from build123d import *

# Parameters (mm, degrees)
SKETCH1_W                   = 14.4272
SKETCH1_H                   = 11.43
CUT_EXTRUDE1_DEPTH          = 22.666423328
CUT_EXTRUDE2_DEPTH          = 22.666423328
CUT_EXTRUDE3_DEPTH          = 22.666423328
CUT_EXTRUDE4_DEPTH          = 22.666423328
CUT_EXTRUDE5_DEPTH          = 22.666423328
CUT_EXTRUDE6_DEPTH          = 22.666423328
CUT_EXTRUDE7_DEPTH          = 22.666423328
CUT_EXTRUDE8_DEPTH          = 22.666423328
CUT_EXTRUDE9_DEPTH          = 22.666423328
CUT_EXTRUDE10_DEPTH         = 22.666423328
CUT_EXTRUDE11_DEPTH         = 22.666423328
CUT_EXTRUDE12_DEPTH         = 22.589197779
CUT_EXTRUDE13_DEPTH         = 22.589197779
CUT_EXTRUDE14_DEPTH         = 22.589197779
CUT_EXTRUDE15_DEPTH         = 22.589197779
CUT_EXTRUDE16_DEPTH         = 22.511694997
F_1_4_0_25_DIAMETER_HOLE1_D = 12.7


with BuildPart() as part:
    # Sketch1 → Revolve1 (revolve)
    with BuildSketch(Plane(origin=(0, 0, 0), x_dir=(-1, 0, 0), z_dir=(0, 0, -1)), mode=Mode.PRIVATE) as revolve1_sk:
        with Locations((-7.2136, 5.715)):
            Rectangle(SKETCH1_W, SKETCH1_H)
    revolve(revolve1_sk.sketch.rotate(Axis((14.4272, 0, 0), (-1, 0, 0)), 270), axis=Axis((14.4272, 0, 0), (-1, 0, 0)))

    # Sketch2 → Cut-Extrude1 (cut, through all)
    with BuildSketch(Plane(origin=(14.4272, 0, 0), x_dir=(0, 0, -1), z_dir=(1, 0, 0))):
        with BuildLine():
            ThreePointArc((9.270604538, 6.685865052), (8.082230509, 8.082230509), (6.685865052, 9.270604538))
            ThreePointArc((6.685865052, 9.270604538), (6.338531077, 7.823071544), (5.493243318, 6.597722098))
            ThreePointArc((5.493243318, 6.597722098), (6.070653138, 6.070653138), (6.597722098, 5.493243318))
            ThreePointArc((6.597722098, 5.493243318), (7.823071544, 6.338531077), (9.270604538, 6.685865052))
        make_face()
    extrude(amount=-CUT_EXTRUDE1_DEPTH, mode=Mode.SUBTRACT)

    # Sketch3 → Cut-Extrude2 (cut, through all)
    with BuildSketch(Plane(origin=(14.4272, 0, 0), x_dir=(0, 0, -1), z_dir=(1, 0, 0))):
        with BuildLine():
            ThreePointArc((11.123491573, 2.629227114), (10.559943057, 4.374071632), (9.724640644, 6.006352))
            ThreePointArc((9.724640644, 6.006352), (8.849798999, 4.801924852), (7.599934007, 3.9933272))
            ThreePointArc((7.599934007, 3.9933272), (7.931690563, 3.285413804), (8.197673616, 2.550256131))
            ThreePointArc((8.197673616, 2.550256131), (9.65322651, 2.862279258), (11.123491573, 2.629227114))
        make_face()
    extrude(amount=-CUT_EXTRUDE2_DEPTH, mode=Mode.SUBTRACT)

    # Sketch4 → Cut-Extrude3 (cut, through all)
    with BuildSketch(Plane(origin=(14.4272, 0, 0), x_dir=(0, 0, -1), z_dir=(1, 0, 0))):
        with BuildLine():
            ThreePointArc((11.282927851, -1.827686818), (11.43, 0), (11.282927851, 1.827686818))
            ThreePointArc((11.282927851, 1.827686818), (10.013765246, 1.049728631), (8.549603637, 0.780984435))
            ThreePointArc((8.549603637, 0.780984435), (8.5852, 0), (8.549603637, -0.780984435))
            ThreePointArc((8.549603637, -0.780984435), (10.013765246, -1.049728631), (11.282927851, -1.827686818))
        make_face()
    extrude(amount=-CUT_EXTRUDE3_DEPTH, mode=Mode.SUBTRACT)

    # Sketch5 → Cut-Extrude4 (cut, through all)
    with BuildSketch(Plane(origin=(14.4272, 0, 0), x_dir=(0, 0, -1), z_dir=(1, 0, 0))):
        with BuildLine():
            ThreePointArc((9.724640644, -6.006352), (10.559943057, -4.374071632), (11.123491573, -2.629227114))
            ThreePointArc((11.123491573, -2.629227114), (9.65322651, -2.862279258), (8.197673616, -2.550256131))
            ThreePointArc((8.197673616, -2.550256131), (7.931690563, -3.285413804), (7.599934007, -3.9933272))
            ThreePointArc((7.599934007, -3.9933272), (8.849798999, -4.801924852), (9.724640644, -6.006352))
        make_face()
    extrude(amount=-CUT_EXTRUDE4_DEPTH, mode=Mode.SUBTRACT)

    # Sketch6 → Cut-Extrude5 (cut, through all)
    with BuildSketch(Plane(origin=(14.4272, 0, 0), x_dir=(0, 0, -1), z_dir=(1, 0, 0))):
        with BuildLine():
            ThreePointArc((6.685865052, -9.270604538), (8.082230509, -8.082230509), (9.270604538, -6.685865052))
            ThreePointArc((9.270604538, -6.685865052), (7.823071544, -6.338531077), (6.597722098, -5.493243318))
            ThreePointArc((6.597722098, -5.493243318), (6.070653138, -6.070653138), (5.493243318, -6.597722098))
            ThreePointArc((5.493243318, -6.597722098), (6.338531077, -7.823071544), (6.685865052, -9.270604538))
        make_face()
    extrude(amount=-CUT_EXTRUDE5_DEPTH, mode=Mode.SUBTRACT)

    # Sketch7 → Cut-Extrude6 (cut, through all)
    with BuildSketch(Plane(origin=(14.4272, 0, 0), x_dir=(0, 0, -1), z_dir=(1, 0, 0))):
        with BuildLine():
            ThreePointArc((2.629227114, -11.123491573), (4.374071632, -10.559943057), (6.006352, -9.724640644))
            ThreePointArc((6.006352, -9.724640644), (4.801924852, -8.849798999), (3.9933272, -7.599934007))
            ThreePointArc((3.9933272, -7.599934007), (3.285413804, -7.931690563), (2.550256131, -8.197673616))
            ThreePointArc((2.550256131, -8.197673616), (2.862279258, -9.65322651), (2.629227114, -11.123491573))
        make_face()
    extrude(amount=-CUT_EXTRUDE6_DEPTH, mode=Mode.SUBTRACT)

    # Sketch8 → Cut-Extrude7 (cut, through all)
    with BuildSketch(Plane(origin=(14.4272, 0, 0), x_dir=(0, 0, -1), z_dir=(1, 0, 0))):
        with BuildLine():
            ThreePointArc((-1.827686818, -11.282927851), (0, -11.43), (1.827686818, -11.282927851))
            ThreePointArc((1.827686818, -11.282927851), (1.049728631, -10.013765246), (0.780984435, -8.549603637))
            ThreePointArc((0.780984435, -8.549603637), (0, -8.5852), (-0.780984435, -8.549603637))
            ThreePointArc((-0.780984435, -8.549603637), (-1.049728631, -10.013765246), (-1.827686818, -11.282927851))
        make_face()
    extrude(amount=-CUT_EXTRUDE7_DEPTH, mode=Mode.SUBTRACT)

    # Sketch9 → Cut-Extrude8 (cut, through all)
    with BuildSketch(Plane(origin=(14.4272, 0, 0), x_dir=(0, 0, -1), z_dir=(1, 0, 0))):
        with BuildLine():
            ThreePointArc((-6.006352, -9.724640644), (-4.374071632, -10.559943057), (-2.629227114, -11.123491573))
            ThreePointArc((-2.629227114, -11.123491573), (-2.862279258, -9.65322651), (-2.550256131, -8.197673616))
            ThreePointArc((-2.550256131, -8.197673616), (-3.285413804, -7.931690563), (-3.9933272, -7.599934007))
            ThreePointArc((-3.9933272, -7.599934007), (-4.801924852, -8.849798999), (-6.006352, -9.724640644))
        make_face()
    extrude(amount=-CUT_EXTRUDE8_DEPTH, mode=Mode.SUBTRACT)

    # Sketch10 → Cut-Extrude9 (cut, through all)
    with BuildSketch(Plane(origin=(14.4272, 0, 0), x_dir=(0, 0, -1), z_dir=(1, 0, 0))):
        with BuildLine():
            ThreePointArc((-9.270604538, -6.685865052), (-8.082230509, -8.082230509), (-6.685865052, -9.270604538))
            ThreePointArc((-6.685865052, -9.270604538), (-6.338531077, -7.823071544), (-5.493243318, -6.597722098))
            ThreePointArc((-5.493243318, -6.597722098), (-6.070653138, -6.070653138), (-6.597722098, -5.493243318))
            ThreePointArc((-6.597722098, -5.493243318), (-7.823071544, -6.338531077), (-9.270604538, -6.685865052))
        make_face()
    extrude(amount=-CUT_EXTRUDE9_DEPTH, mode=Mode.SUBTRACT)

    # Sketch11 → Cut-Extrude10 (cut, through all)
    with BuildSketch(Plane(origin=(14.4272, 0, 0), x_dir=(0, 0, -1), z_dir=(1, 0, 0))):
        with BuildLine():
            ThreePointArc((-11.123491573, -2.629227114), (-10.559943057, -4.374071632), (-9.724640644, -6.006352))
            ThreePointArc((-9.724640644, -6.006352), (-8.849798999, -4.801924852), (-7.599934007, -3.9933272))
            ThreePointArc((-7.599934007, -3.9933272), (-7.931690563, -3.285413804), (-8.197673616, -2.550256131))
            ThreePointArc((-8.197673616, -2.550256131), (-9.65322651, -2.862279258), (-11.123491573, -2.629227114))
        make_face()
    extrude(amount=-CUT_EXTRUDE10_DEPTH, mode=Mode.SUBTRACT)

    # Sketch12 → Cut-Extrude11 (cut, through all)
    with BuildSketch(Plane(origin=(14.4272, 0, 0), x_dir=(0, 0, -1), z_dir=(1, 0, 0))):
        with BuildLine():
            ThreePointArc((-11.282927851, 1.827686818), (-11.43, 0), (-11.282927851, -1.827686818))
            ThreePointArc((-11.282927851, -1.827686818), (-10.013765246, -1.049728631), (-8.549603637, -0.780984435))
            ThreePointArc((-8.549603637, -0.780984435), (-8.5852, 0), (-8.549603637, 0.780984435))
            ThreePointArc((-8.549603637, 0.780984435), (-10.013765246, 1.049728631), (-11.282927851, 1.827686818))
        make_face()
    extrude(amount=-CUT_EXTRUDE11_DEPTH, mode=Mode.SUBTRACT)

    # Sketch13 → Cut-Extrude12 (cut, through all)
    with BuildSketch(Plane(origin=(14.4272, 0, 0), x_dir=(0, 0, -1), z_dir=(1, 0, 0))):
        with BuildLine():
            ThreePointArc((-9.724640644, 6.006352), (-10.559943057, 4.374071632), (-11.123491573, 2.629227114))
            ThreePointArc((-11.123491573, 2.629227114), (-9.65322651, 2.862279258), (-8.197673616, 2.550256131))
            ThreePointArc((-8.197673616, 2.550256131), (-7.931690563, 3.285413804), (-7.599934007, 3.9933272))
            ThreePointArc((-7.599934007, 3.9933272), (-8.849798999, 4.801924852), (-9.724640644, 6.006352))
        make_face()
    extrude(amount=-CUT_EXTRUDE12_DEPTH, mode=Mode.SUBTRACT)

    # Sketch14 → Cut-Extrude13 (cut, through all)
    with BuildSketch(Plane(origin=(14.4272, 0, 0), x_dir=(0, 0, -1), z_dir=(1, 0, 0))):
        with BuildLine():
            ThreePointArc((-6.685865052, 9.270604538), (-8.082230509, 8.082230509), (-9.270604538, 6.685865052))
            ThreePointArc((-9.270604538, 6.685865052), (-7.823071544, 6.338531077), (-6.597722098, 5.493243318))
            ThreePointArc((-6.597722098, 5.493243318), (-6.070653138, 6.070653138), (-5.493243318, 6.597722098))
            ThreePointArc((-5.493243318, 6.597722098), (-6.338531077, 7.823071544), (-6.685865052, 9.270604538))
        make_face()
    extrude(amount=-CUT_EXTRUDE13_DEPTH, mode=Mode.SUBTRACT)

    # Sketch15 → Cut-Extrude14 (cut, through all)
    with BuildSketch(Plane(origin=(14.4272, 0, 0), x_dir=(0, 0, -1), z_dir=(1, 0, 0))):
        with BuildLine():
            ThreePointArc((-2.629227114, 11.123491573), (-4.374071632, 10.559943057), (-6.006352, 9.724640644))
            ThreePointArc((-6.006352, 9.724640644), (-4.801924852, 8.849798999), (-3.9933272, 7.599934007))
            ThreePointArc((-3.9933272, 7.599934007), (-3.285413804, 7.931690563), (-2.550256131, 8.197673616))
            ThreePointArc((-2.550256131, 8.197673616), (-2.862279258, 9.65322651), (-2.629227114, 11.123491573))
        make_face()
    extrude(amount=-CUT_EXTRUDE14_DEPTH, mode=Mode.SUBTRACT)

    # Sketch16 → Cut-Extrude15 (cut, through all)
    with BuildSketch(Plane(origin=(14.4272, 0, 0), x_dir=(0, 0, -1), z_dir=(1, 0, 0))):
        with BuildLine():
            ThreePointArc((1.827686818, 11.282927851), (0, 11.43), (-1.827686818, 11.282927851))
            ThreePointArc((-1.827686818, 11.282927851), (-1.049728631, 10.013765246), (-0.780984435, 8.549603637))
            ThreePointArc((-0.780984435, 8.549603637), (0, 8.5852), (0.780984435, 8.549603637))
            ThreePointArc((0.780984435, 8.549603637), (1.049728631, 10.013765246), (1.827686818, 11.282927851))
        make_face()
    extrude(amount=-CUT_EXTRUDE15_DEPTH, mode=Mode.SUBTRACT)

    # Sketch17 → Cut-Extrude16 (cut, through all)
    with BuildSketch(Plane(origin=(14.4272, 0, 0), x_dir=(0, 0, -1), z_dir=(1, 0, 0))):
        with BuildLine():
            ThreePointArc((6.006352, 9.724640644), (4.374071632, 10.559943057), (2.629227114, 11.123491573))
            ThreePointArc((2.629227114, 11.123491573), (2.862279258, 9.65322651), (2.550256131, 8.197673616))
            ThreePointArc((2.550256131, 8.197673616), (3.285413804, 7.931690563), (3.9933272, 7.599934007))
            ThreePointArc((3.9933272, 7.599934007), (4.801924852, 8.849798999), (6.006352, 9.724640644))
        make_face()
    extrude(amount=-CUT_EXTRUDE16_DEPTH, mode=Mode.SUBTRACT)

    # 1/4 (0.25) Diameter Hole1 (through all)
    with Locations(Plane(origin=(14.4272, 0, 0), x_dir=(0, 0, -1), z_dir=(1, 0, 0))):
        with Locations((0, 0)):
            Hole(F_1_4_0_25_DIAMETER_HOLE1_D / 2)


solid = part.part
The model under review builds one solid part; all positions refer to its coordinate system, in mm. A direction names the side the tool comes from. Coordinates: 2 decimals unless noted, no trailing zeros. Write each loop counter-clockwise with the first axis right and the second up, starting at its lowest first coordinate (ties: lowest second). Pieces come first, ordered by that corner, then holes. Notation, with made-up numbers: (62, 32.25) - (104, 32.25) arc R22 cw to (104, 63.25) - close; hole circle Ø9 at (5.25, -3.5). An arc over 180 degrees is marked (long way). Answer as CSV lines item,"result".
(1) Mouldability with a two-part tool opening along Y and no side actions: class faces 1 (the cylindrical face through (7.113, 2.224, 11.211)), 2 (the cylindrical face through (7.315, -2.863, -9.674)), 3 (the flat face through (14.427, 5, 5)) as pulls with the +Y half, pulls with the -Y half, needs draft (parallel to the pull), parting line crosses it, or undercut.
Data:
face 1,"pulls with the +Y half"
face 2,"undercut"
face 3,"needs draft"
(2) For line 1 along Y through (x, z) = (6.5, 0); line 2 along Y through (x, z) = (10.75, 9); line 3 along Y through (x, z) = (6.75, -4.5), list the stretches that pass through material, from the lowest coordinate up. Write a range as [from, to].
Data:
line 1,"y = [-8.59, -6.35], [6.35, 8.59]"
line 2,"y = [-6.66, -4.95], [-2.79, -0.8], [0.8, 2.79], [4.95, 6.66]"
line 3,"y = [-8.49, -4.48], [4.48, 8.49]"
(3) We need section C-C (y = 7). Give the boundary of the cut face in (x, z).
Data:
outline,"(0, -5.85) - (14.43, -5.85) - (14.43, 5.85) - (0, 5.85) - close"
(4) We need section A-A (y = 0). Give the boundary of the cut face in (x, z), plus the area to 3 significant figures.
Data:
outline,"(0, -8.59) - (14.43, -8.59) - (14.43, -6.35) - (0, -6.35) - close; (0, 6.35) - (14.43, 6.35) - (14.43, 8.59) - (0, 8.59) - close"
area,"64.5 mm2"
(5) Tool access review of faces 4 (the cylindrical face through (7.315, 3.296, -7.927)), 5 (the cylindrical face through (7.315, -0.011, 8.585)): name each direction out of +Z, -Z, +X, -X, +Y, -Y from which nothing blocks a thin tool from reaching the whole face with its end or side.
Data:
face 4,"+X, -X"
face 5,"+Z, +X, -X"
(6) Clearance check with flat-ended pins moving along their axes: pin 1 Ø1 at (y, z) = (-3.5, -7.5) entering from -X; pin 2 Ø1 at (x, y) = (11, 4) entering from +Z; pin 3 Ø1 at (x, z) = (3, 3.5) entering from -Y; pin 4 Ø1 at (x, z) = (2, 2.5) entering from -Y. State where each tip first meets the part, or that it passes through.
Data:
pin 1,"stops at x = 0"
pin 2,"stops at z = 8.49"
pin 3,"stops at y = -8.04"
pin 4,"stops at y = -11.25"
